from build123d import *

# Parameters (mm, degrees)
F0_R     = 7.874
F1_DEPTH = 10.922
F0_W     = 52.578
F0_H     = 10.922
F2_DEPTH = 33.528
F3_SIZE2 = 16.571107
F3_SIZE  = 28.702
F5_DEPTH = 25.4


with BuildPart() as f1:
    # F0 (on Front) → F1 (new body)
    with BuildSketch(Plane.XZ):
        Polygon((-63.5, 27.104102), (-63.5, 17.706102), (-52.578, 17.706102), (-52.578, -22.171898), (0, -22.171898), (0, -33.093898), (50.8, -33.093898), (50.8, 4.984896), (-31.75, 27.104102), align=None)
        with Locations((31.75, -14.043898)):
            Circle(F0_R, mode=Mode.SUBTRACT)
    extrude(amount=F1_DEPTH)

    # F0 (on Front) → F2 (join)
    with BuildSketch(Plane.XZ):
        Polygon((-63.5, 17.706102), (-63.5, -33.093898), (-52.578, -33.093898), (-52.578, -22.171898), (-52.578, 17.706102), align=None)
        with Locations((-26.289, -27.632898)):
            Rectangle(F0_W, F0_H)
    extrude(amount=F2_DEPTH)

    # F3
    f3_edges = [f1.edges().sort_by_distance(p)[0] for p in [
        (-58.039, -33.528, 17.706102),
    ]]
    chamfer(f3_edges, length=F3_SIZE, length2=F3_SIZE2)

    # F4 (on face) → F5 (cut)
    with BuildSketch(Plane.XY.offset(-22.171898)):
        Polygon((0, -10.922), (-52.578, -33.528), (0, -33.528), align=None)
    extrude(amount=-F5_DEPTH, mode=Mode.SUBTRACT)


solid = f1.part
Input: part model. Units: mm. Frame: model coordinates. A direction names the side the tool comes from. Coordinates: 2 decimals unless noted, no trailing zeros. Order: outer loops, then holes, each group sorted by start corner. A loop starts at its lowest first (then second) coordinate and runs counter-clockwise, first axis right, second up. Notation, with made-up numbers: M -36,-24 L 2,-24 A18 cw 2,8 Z; hole C 30,63.5 d3. An arc over 180 degrees is marked long. One line per question, with ' | ' between items.
Item 1: Section D-D (z = 15.5). Output: boundary loops of the cut face in (x, y).
Geometry results:
outline: M -63.5,-18.23 L -52.58,-18.23 L -52.58,-10.92 L 11.56,-10.92 L 11.56,0 L -63.5,0 Z
Item 2: Ray query, line 1 along Y through (x, z) = (-49, 3); line 2 along Z through (x, y) = (31.75, -3.75); line 3 along X through (y, z) = (-4.5, -8.5). Return the intervals inside material, ascending.
Geometry results:
line 1: y = -10.92 to 0 | line 2: z = -33.09 to -21.92, -6.17 to 10.09 | line 3: x = -63.5 to 26.16, 37.34 to 50.8
Item 3: Pin query (flat end, axial travel): pin 1 (3 mm diameter, centred on x = 0.5, y = -14, fed in from -Z); pin 2 (10 mm diameter, centred on x = -40, z = -16, fed in from -Y); pin 3 (1.8 mm diameter, centred on x = -59.5, y = -14.5, fed in from +Z); pin 4 (4 mm diameter, centred on x = 38.5, y = -4, fed in from +Z). Return the tip coordinate at first contact, or that it passes through.
Geometry results:
pin 1: passes through | pin 2: stops at y = -10.92 | pin 3: stops at z = 17.71 | pin 4: stops at z = 8.82
Item 4: Section C-C (x = -44). Output: boundary loops of the cut face in (y, z).
Geometry results:
outline: M -29.84,-33.09 L 0,-33.09 L 0,27.1 L -10.92,27.1 L -10.92,-22.17 L -29.84,-22.17 Z
Item 5: Section A-A (x = 31.75). Output: boundary loops of the cut face in (y, z), then the cut area to 3 significant figures.
Geometry results:
outline: M -10.92,-33.09 L 0,-33.09 L 0,-21.92 L -10.92,-21.92 Z; M -10.92,-6.17 L 0,-6.17 L 0,10.09 L -10.92,10.09 Z | area: 300 mm^2
Item 6: Section B-B (z = -9.5). Output: boundary loops of the cut face in (x, y).
Geometry results:
outline: M -63.5,-32.66 L -52.58,-32.66 L -52.58,-10.92 L 25.32,-10.92 L 25.32,0 L -63.5,0 Z; M 38.18,-10.92 L 50.8,-10.92 L 50.8,0 L 38.18,0 Z
Item 7: Draft query along Z for faces 1 (the cylindrical face through (25.501, -5.385, -18.835)), 2 (the flat face through (10.1, -5.38, 15.89)), 3 (the flat face through (50.8, -5, -14)). Return one class per face: released by +Z, released by -Z, zero draft, split by the parting line, or undercut.
Geometry results:
face 1: undercut | face 2: released by +Z | face 3: zero draft
Item 8: Reachability of faces 4 (the flat face through (-63.5, -13, -9)), 5 (the flat face through (-58, -14, 17.706)), 6 (the flat face through (-52.578, -20, -7)) from +Z, -Z, +X, -X, +Y, -Y: full face, straight path, thin tool, end or side. Return the list, or none.
Geometry results:
face 4: +Z, -Z, -X, +Y, -Y | face 5: +Z, +X, -X, -Y | face 6: +Z, +X, -Y
